Build history of the part. All positions in model axes, mm. Face numbers are marked on the shaded views. Round coordinates to 2 decimals unless told otherwise and drop trailing zeros. Write each loop counter-clockwise with the first axis right and the second up, starting at its lowest first coordinate (ties: lowest second). Pieces come first, ordered by that corner, then holes. Notation, with made-up numbers: (72.5, 85) -> (106.5, 85) arc R11 ccw to (106.5, 92) -> close; hole circle Ø8 at (44, -9.5). An arc over 180 degrees is marked (long way). One line per question, with ' | ' between items.
from build123d import *

# Parameters (mm, degrees)
EXTRUDE_1_DEPTH          = 25
CUT_EXTRUDE_1_DEPTH      = 25
CUT_EXTRUDE_1_DEPTH_BACK = 25
SKETCH_2_R               = 1.4
SKETCH_2_W               = 8.931793576
SKETCH_2_H               = 6.25
SKETCH_2_H_2             = 7.571808546
CHAMFER_1_SIZE           = 0.8


with BuildPart() as part:
    # Эскиз1 → Вытянуть1 (new body)
    with BuildSketch(Plane.XY):
        with BuildLine():
            Line((0, 0), (13.5, 0))
            Line((13.5, 0), (13.5, 1))
            Line((13.5, 1), (0, 1))
            ThreePointArc((0, 1), (-0.387298335, 3.949137675), (0.748331477, 1.2))
            Line((0.748331477, 1.2), (2.13541565, 1.2))
            ThreePointArc((2.13541565, 1.2), (-1.224744871, 4.679449472), (0, 0))
        make_face()
    extrude(amount=EXTRUDE_1_DEPTH)

    # Эскиз2 → Вырез-Вытянуть1 (cut, two sides: drawn at the far end of the back side and taken through both)
    with BuildSketch(Plane(origin=(0, 1, 0), x_dir=(-1, 0, 0), z_dir=(0, 1, 0)).offset(-CUT_EXTRUDE_1_DEPTH_BACK)):
        with Locations((-8.5, 20)):
            Circle(SKETCH_2_R)
        with Locations((-8.5, 5)):
            Circle(SKETCH_2_R)
        with Locations((0.465896788, 15.625)):
            Rectangle(SKETCH_2_W, SKETCH_2_H)
        with Locations((0.465896788, 2.464095727)):
            Rectangle(SKETCH_2_W, SKETCH_2_H_2)
    extrude(amount=CUT_EXTRUDE_1_DEPTH + CUT_EXTRUDE_1_DEPTH_BACK, mode=Mode.SUBTRACT)

    # Фаска1
    chamfer_1_edges = [part.edges().sort_by_distance(p)[0] for p in [
        (9.9, 1, 20),
        (9.9, 1, 5),
    ]]
    chamfer(chamfer_1_edges, length=CHAMFER_1_SIZE)


solid = part.part
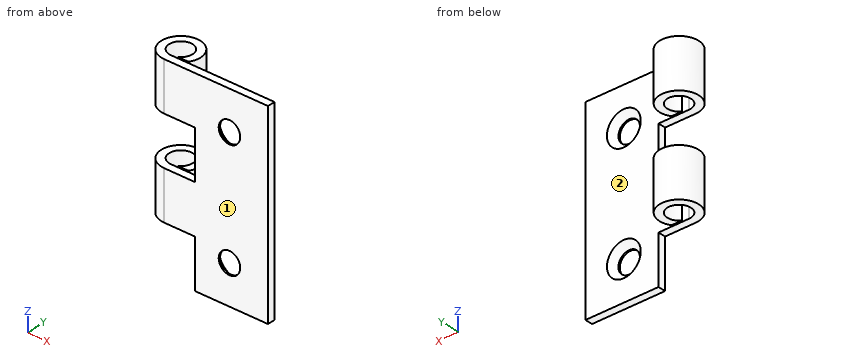
(1) Slice it at C-C (z = 20). Write the cut outline in (x, y), then the cut area to 3 significant figures.
Calculated:
outline: (0, 0) -> (7.1, 0) -> (7.1, 0.2) -> (6.3, 1) -> (0, 1) arc R1.5 cw (long way) to (0.75, 1.2) -> (2.14, 1.2) arc R2.5 ccw (long way) to start; (9.9, 0) -> (13.5, 0) -> (13.5, 1) -> (10.7, 1) -> (9.9, 0.2) -> close | area: 20.9 mm2
(2) Slice it at B-B (x = 8.5). Write the cut outline in (y, z), then the cut area to 3 significant figures.
Calculated:
outline: (0, 0) -> (1, 0) -> (1, 2.8) -> (0.2, 3.6) -> (0, 3.6) -> close; (0, 6.4) -> (0.2, 6.4) -> (1, 7.2) -> (1, 17.8) -> (0.2, 18.6) -> (0, 18.6) -> close; (0, 21.4) -> (0.2, 21.4) -> (1, 22.2) -> (1, 25) -> (0, 25) -> close | area: 18.1 mm2
(3) Slice it at A-A (y = 2.5). Write the cut outline in (x, z), then the cut area to 3 significant figures.
Calculated:
outline: (-2.5, 6.25) -> (-1.5, 6.25) -> (-1.5, 12.5) -> (-2.5, 12.5) -> close; (-2.5, 18.75) -> (-1.5, 18.75) -> (-1.5, 25) -> (-2.5, 25) -> close; (1.5, 6.25) -> (2.5, 6.25) -> (2.5, 12.5) -> (1.5, 12.5) -> close; (1.5, 18.75) -> (2.5, 18.75) -> (2.5, 25) -> (1.5, 25) -> close | area: 25.0 mm2
(4) Mould opens along Y. For the marked faces 1 and 2 say: pulls with the +Y half, pulls with the -Y half, needs draft (parallel to the pull), parting line crosses it, or undercut.
Calculated:
face 1: pulls with the -Y half | face 2: undercut
(5) Slice it at D-D (x = 3). Write the cut outline in (y, z).
Calculated:
outline: (0, 6.25) -> (1, 6.25) -> (1, 12.5) -> (0, 12.5) -> close; (0, 18.75) -> (1, 18.75) -> (1, 25) -> (0, 25) -> close
(6) Wall check: line 1 (Z direction, x = 8.5, y = 0.1); line 2 (Y direction, x = 2, z = 22); line 3 (Z direction, x = 1.75, y = 3.55). Give the ranges that are in metal, low to high. Write a range as from..to.
Calculated:
line 1: 0..3.6, 6.4..18.6, 21.4..25 | line 2: 0..1, 1.2..4 | line 3: 6.25..12.5, 18.75..25
(7) Drop flat-ended pins along their axis: pin 1 (0.5 mm diameter, centred on y = 0.5, z = 15.5, fed in from -X); pin 2 (2.5 mm diameter, centred on x = 0, y = 2.5, fed in from +Z); pin 3 (3 mm diameter, centred on x = 8.5, z = 5, fed in from +Y); pin 4 (2.5 mm diameter, centred on x = 0.5, y = 2, fed in from -Z). Give the stop position or say it passes through.
Calculated:
pin 1: x = 4 | pin 2: through | pin 3: y = 0.3 | pin 4: z = 6.25
